The drawing under review shows one solid part. Ordinate dimensions are in mm from its lowest x, y, z. Round coordinates to 2 decimals unless told otherwise and drop trailing zeros. Write each loop counter-clockwise with the first axis right and the second up, starting at its lowest first coordinate (ties: lowest second). Pieces come first, ordered by that corner, then holes. Notation, with made-up numbers: M 40.5,-36 L 63.5,-36 A12 ccw 63.5,-28 Z; hole C 13,68 d1. An arc over 180 degrees is marked long. Write item = value, one per line. Start each with the question number.
Item 1: Take a section at B-B, the plane z = 22.25. Give the boundary of the cut face in (x, y), plus the area to 3 significant figures.
Item 2: Take a section at C-C, the plane z = 3.5. Give the boundary of the cut face in (x, y).
Item 3: Take a section at A-A, the plane y = 30. Give the boundary of the cut face in (x, z).
Item 4: Take a section at D-D, the plane z = 14. Give the boundary of the cut face in (x, y), plus the area to 3 significant figures.
Item 5: The part is to be moulded in two halves that separate along Y. For the marked faces 1, 2, 3 and 4, say which applies: +Y half, -Y half, draft (parallel to the pull), parting line (faces both ways), or undercut.
Item 6: For pin 1 Ø4 at (x, z) = (35, 25) entering from +Y; pin 2 Ø6 at (x, y) = (30, 7.7) entering from +Z; pin 3 Ø3 at (x, y) = (7.7, 30) entering from -Z; pin 4 Ø12 at (x, z) = (32.5, 22) entering from -Y, all flat-tipped, find the tip position at first contact; note any pin that passes through.
Item 7: To check wall thickness, follow line 1 along Y through (x, z) = (30, 8.25); line 2 along Y through (x, z) = (30, 22.25); line 3 along Z through (x, y) = (15, 13.5). State the ranges of each line that lie inside material, in increasing order.
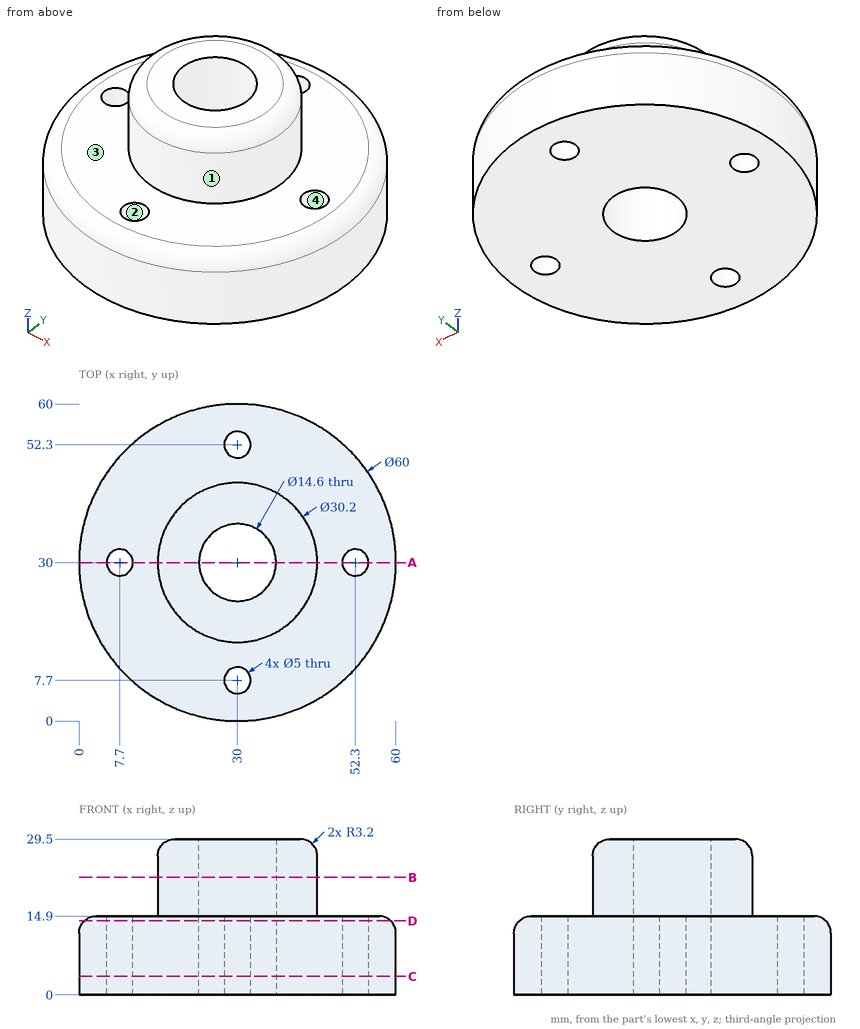
Response values:
q1.outline = C 30,30 d30.2; hole C 30,30 d14.6
q1.area = 549 mm2
q2.outline = C 30,30 d60; hole C 7.7,30 d5; hole C 30,30 d14.6; hole C 30,7.7 d5; hole C 30,52.3 d5; hole C 52.3,30 d5
q3.outline = M 0,0 L 5.2,0 L 5.2,14.9 L 3.2,14.9 A3.2 ccw 0,11.7 Z; M 10.2,0 L 22.7,0 L 22.7,29.5 L 18.1,29.5 A3.2 ccw 14.9,26.3 L 14.9,14.9 L 10.2,14.9 Z; M 37.3,0 L 49.8,0 L 49.8,14.9 L 45.1,14.9 L 45.1,26.3 A3.2 ccw 41.9,29.5 L 37.3,29.5 Z; M 54.8,0 L 60,0 L 60,11.7 A3.2 ccw 56.8,14.9 L 54.8,14.9 Z
q4.outline = C 30,30 d58.05; hole C 7.7,30 d5; hole C 30,30 d14.6; hole C 30,7.7 d5; hole C 30,52.3 d5; hole C 52.3,30 d5
q4.area = 2,400 mm2
q5.face_1 = parting line
q5.face_2 = undercut
q5.face_3 = draft
q5.face_4 = undercut
q6.pin_1 = 44.8
q6.pin_2 = 14.9
q6.pin_3 = through
q6.pin_4 = 14.9
q7.line_1 = 0 to 5.2, 10.2 to 22.7, 37.3 to 49.8, 54.8 to 60
q7.line_2 = 14.9 to 22.7, 37.3 to 45.1
q7.line_3 = 0 to 14.9
